Could you check a few things on this model? Use its own coordinates, in mm. A direction names the side the tool comes from. Give positions to 0.01 mm unless a question says otherwise; leave off trailing zeros. Write each loop counter-clockwise with the first axis right and the second up, starting at its lowest first coordinate (ties: lowest second). Pieces come first, ordered by that corner, then holes. Notation, with made-up numbers: (8, -2) -> (36, -2) arc R19 cw to (36, 25) -> close; hole circle Ø6 at (15, 89). An arc over 180 degrees is marked (long way). One line per question, with ' | ' between items.
Autodesk Fusion 360 part; units mm, degrees
sketch "Skizze1" plane through (0, 0, 0) normal (1, 0, 0) x (0, 1, 0)
  line L0 (0, 0) -> (0, 17.0455) construction
  line L1 (0, 0) -> (-3.9, 0)
  line L2 (-3.9, 0) -> (-3.9, 3.9)
  line L3 (-3.9, 3.9) -> (-7.15, 3.9)
  line L4 (-7.15, 3.9) -> (-7.15, 9.9)
  line L5 (-7.15, 9.9) -> (0, 9.9)
  line L6 (0, 0) -> (3.9, 0)
  line L7 (3.9, 0) -> (3.9, 3.9)
  line L8 (3.9, 3.9) -> (7.15, 3.9)
  line L9 (7.15, 3.9) -> (7.15, 9.9)
  line L10 (7.15, 9.9) -> (0, 9.9)
  dimension "d2" = 14.3
  dimension "d4" = 3.9
  dimension "d5" = 7.8
  dimension "d17" = 6
extrude "Extrusion1" add sketch "Skizze1" along normal blind 25
sketch "Skizze2" plane through (0, 0, 9.9) normal (0, 0, 1) x (-1, 0, 0)
  line L0 (0, -7.15) -> (0, 7.15)
  line L1 (0, 7.15) -> (-25, 7.15)
  line L2 (-25, 7.15) -> (-25, -7.15)
  line L3 (-25, -7.15) -> (0, -7.15)
  line L4 (-12.5, -7.15) -> (-12.5, 7.15)
  circle A0 centre (-20, 0) radius 1.65
  line L5 (-17.1, 1.6743) -> (-20, 3.3486)
  line L6 (-20, 3.3486) -> (-22.9, 1.6743)
  line L7 (-22.9, 1.6743) -> (-22.9, -1.6743)
  line L8 (-22.9, -1.6743) -> (-20, -3.3486)
  line L9 (-20, -3.3486) -> (-17.1, -1.6743)
  line L10 (-17.1, -1.6743) -> (-17.1, 1.6743)
  line L11 (-12.5, 0) -> (-20, 0) construction
  line L12 (-7.9, -1.6743) -> (-7.9, 1.6743)
  line L13 (-5, 3.3486) -> (-2.1, 1.6743)
  line L14 (-2.1, -1.6743) -> (-5, -3.3486)
  line L15 (-5, -3.3486) -> (-7.9, -1.6743)
  line L16 (-7.9, 1.6743) -> (-5, 3.3486)
  line L17 (-2.1, 1.6743) -> (-2.1, -1.6743)
  circle A1 centre (-5, 0) radius 1.65
  point P0 (-20, 0)
  point P1 (-5, 0)
  point P2 (-5, 0)
  dimension "d8" = 3.3
  dimension "d9" = 5.8
  dimension "d10" = 15
extrude "Extrusion2" cut sketch "Skizze2" against normal through all contours A0 | A1
extrude "Extrusion3" cut sketch "Skizze2" against normal blind 3.2 contours L5 L6 L7 L8 L9 L10 | L12 L13 L14 L15 L16 L17
chamfer "Fase1" distance 0.3 angle 45 4 edges at (6.5383, 0.5967, 0) (21.5383, 0.5967, 0) (6.5383, 0.5967, 6.7) (21.5383, 0.5967, 6.7)
chamfer "Fase1" distance 0.5 angle 45 22 edges at (0, 7.15, 6.9) (0, -7.15, 6.9) (25, -7.15, 6.9) (25, 7.15, 6.9) (25, 3.9, 1.95) (25, -3.9, 1.95) (0, -3.9, 1.95) (0, 3.9, 1.95) (12.5, 7.15, 9.9) (12.5, -7.15, 9.9) (12.5, 7.15, 3.9) (12.5, -7.15, 3.9) (12.5, 3.9, 0) (12.5, -3.9, 0) (25, -5.525, 3.9) (25, 5.525, 3.9) (0, 5.525, 3.9) (0, -5.525, 3.9) (0, 0, 0) (25, 0, 0) (25, 0, 9.9) (0, 0, 9.9)
chamfer "Fase1" distance 0.3 angle 45 12 edges at (3.55, 2.5115, 9.9) (6.45, 2.5115, 9.9) (7.9, 0, 9.9) (6.45, -2.5115, 9.9) (3.55, -2.5115, 9.9) (2.1, 0, 9.9) (17.1, 0, 9.9) (18.55, 2.5115, 9.9) (21.45, 2.5115, 9.9) (22.9, 0, 9.9) (21.45, -2.5115, 9.9) (18.55, -2.5115, 9.9)
Q1. Will these pins go through, and if not, where does the flat tip stop? pin 1 (2.5 mm diameter, centred on x = 20, y = 0, fed in from +Z); pin 2 (3 mm diameter, centred on x = 12.5, y = 6, fed in from -Z); pin 3 (1 mm diameter, centred on x = 10, z = 1.5, fed in from -Y); pin 4 (1 mm diameter, centred on x = 15.5, y = 4, fed in from -Z).
Answer below:
pin 1: passes through | pin 2: stops at z = 3.9 | pin 3: stops at y = -3.9 | pin 4: stops at z = 0.1
Q2. If I drill on line 1 along X through (y, z) = (0, 2.75); line 2 along X through (y, z) = (0.5, 7.75); line 3 along Y through (x, z) = (5, 5.25), over which ranges is the centre line in solid material (lowest first)?
Answer below:
line 1: x = 0 to 3.35, 6.65 to 18.35, 21.65 to 25 | line 2: x = 0 to 2.1, 7.9 to 17.1, 22.9 to 25 | line 3: y = -7.15 to -1.65, 1.65 to 7.15
Q3. On a 3-axis mill with a long thin cutter (end or side, diameter ignored), from which of +Z, -Z, +X, -X, +Y, -Y can I reach the whole of each face in a straight line? I mean faces 5 (the flat face through (22, 1, 6.7)), 6 (the flat face through (25, 0, 6)). Say none if no direction works.
Answer below:
face 5: +Z | face 6: +Z, -Z, +X, +Y, -Y
Q4. Imagine slicing it at D-D on y = 0. Count the separate pieces of the cut face and the enclosed holes in it, and give its area (3 significant figures).
Answer below:
separate pieces: 3 | enclosed holes: 0 | area: 165 mm^2
Q5. Imagine slicing it at A-A on z = 8.5. Please give me the cut outline in (x, y), and give its area (3 significant figures).
Answer below:
outline: (0, -6.65) -> (0.5, -7.15) -> (24.5, -7.15) -> (25, -6.65) -> (25, 6.65) -> (24.5, 7.15) -> (0.5, 7.15) -> (0, 6.65) -> close; hole (2.1, -1.67) -> (5, -3.35) -> (7.9, -1.67) -> (7.9, 1.67) -> (5, 3.35) -> (2.1, 1.67) -> close; hole (17.1, -1.67) -> (20, -3.35) -> (22.9, -1.67) -> (22.9, 1.67) -> (20, 3.35) -> (17.1, 1.67) -> close | area: 299 mm^2
Q6. Imagine slicing it at B-B on y = -5. Please give me the cut outline in (x, z).
Answer below:
outline: (0, 4.4) -> (0.5, 3.9) -> (24.5, 3.9) -> (25, 4.4) -> (25, 9.4) -> (24.5, 9.9) -> (0.5, 9.9) -> (0, 9.4) -> close
Q7. Imagine slicing it at C-C on x = 9.25. Please give me the cut outline in (y, z).
Answer below:
outline: (-7.15, 4.4) -> (-6.65, 3.9) -> (-3.9, 3.9) -> (-3.9, 0.5) -> (-3.4, 0) -> (3.4, 0) -> (3.9, 0.5) -> (3.9, 3.9) -> (6.65, 3.9) -> (7.15, 4.4) -> (7.15, 9.4) -> (6.65, 9.9) -> (-6.65, 9.9) -> (-7.15, 9.4) -> close
Q8. If we mould it in two halves opening along Y, with no side actions, what happens to faces 1 (the flat face through (12, -3.9, 2)), 2 (the flat face through (12, -5, 3.9)), 3 (the flat face through (3.53, 2.5, 8.17)), 4 (the flat face through (6.47, -2.5, 8.17))? For each: +Y half, -Y half, draft (parallel to the pull), parting line (faces both ways), or undercut.
Answer below:
face 1: -Y half | face 2: draft | face 3: undercut | face 4: undercut
